from build123d import *

# Parameters (mm, degrees)
F0_R     = 6.45
F0_R_2   = 11.175
F1_DEPTH = 7
F2_R     = 3


with BuildPart() as f1:
    # F0 (on Top) → F1 (new body)
    with BuildSketch(Plane.XY):
        with BuildLine():
            ThreePointArc((9.599923, 11.660709), (13.65884, 6.447227), (15.103995, 0))
            ThreePointArc((15.103995, 0), (13.65884, -6.447227), (9.599923, -11.660709))
            ThreePointArc((9.599923, -11.660709), (14.033897, -12.989573), (18.629101, -13.546434))
            ThreePointArc((18.629101, -13.546434), (32.744063, -10.165399), (43.103995, 0))
            ThreePointArc((43.103995, 0), (32.744063, 10.165399), (18.629101, 13.546434))
            ThreePointArc((18.629101, 13.546434), (14.033897, 12.989573), (9.599923, 11.660709))
        make_face()
        with Locations((28.517951, 0)):
            Circle(F0_R, mode=Mode.SUBTRACT)
        with BuildLine():
            ThreePointArc((-9.599923, 11.660709), (0, 15.103995), (9.599923, 11.660709))
            ThreePointArc((9.599923, 11.660709), (14.033897, 12.989573), (18.629101, 13.546434))
            ThreePointArc((18.629101, 13.546434), (7.362471, 16.703494), (0, 25.797338))
            ThreePointArc((0, 25.797338), (-7.362471, 16.703494), (-18.629101, 13.546434))
            ThreePointArc((-18.629101, 13.546434), (-14.033897, 12.989573), (-9.599923, 11.660709))
        make_face()
        with BuildLine():
            ThreePointArc((18.629101, -13.546434), (14.033897, -12.989573), (9.599923, -11.660709))
            ThreePointArc((9.599923, -11.660709), (0, -15.103995), (-9.599923, -11.660709))
            ThreePointArc((-9.599923, -11.660709), (-14.033897, -12.989573), (-18.629101, -13.546434))
            ThreePointArc((-18.629101, -13.546434), (-7.362471, -16.703494), (0, -25.797338))
            ThreePointArc((0, -25.797338), (7.362471, -16.703494), (18.629101, -13.546434))
        make_face()
        with BuildLine():
            ThreePointArc((-9.599923, -11.660709), (-15.103995, 0), (-9.599923, 11.660709))
            ThreePointArc((-9.599923, 11.660709), (-14.033897, 12.989573), (-18.629101, 13.546434))
            ThreePointArc((-18.629101, 13.546434), (-32.744063, 10.165399), (-43.103995, 0))
            ThreePointArc((-43.103995, 0), (-32.744063, -10.165399), (-18.629101, -13.546434))
            ThreePointArc((-18.629101, -13.546434), (-14.033897, -12.989573), (-9.599923, -11.660709))
        make_face()
        with Locations((-28.517951, 0)):
            Circle(F0_R, mode=Mode.SUBTRACT)
        with BuildLine():
            ThreePointArc((9.599923, -11.660709), (13.65884, -6.447227), (15.103995, 0))
            ThreePointArc((15.103995, 0), (13.65884, 6.447227), (9.599923, 11.660709))
            ThreePointArc((9.599923, 11.660709), (0, 15.103995), (-9.599923, 11.660709))
            ThreePointArc((-9.599923, 11.660709), (-15.103995, 0), (-9.599923, -11.660709))
            ThreePointArc((-9.599923, -11.660709), (0, -15.103995), (9.599923, -11.660709))
        make_face()
        Circle(F0_R_2, mode=Mode.SUBTRACT)
    extrude(amount=F1_DEPTH)

    # F2
    f2_edges = [f1.edges().sort_by_distance(p)[0] for p in [
        (7.362471, -16.703494, 7),
        (32.744063, -10.165399, 7),
        (32.744063, 10.165399, 7),
        (7.362471, 16.703494, 7),
        (-7.362471, 16.703494, 7),
        (-32.744063, -10.165399, 7),
        (-7.362471, -16.703494, 7),
        (-32.744063, 10.165399, 7),
        (7.362471, -16.703494, 0),
        (32.744063, -10.165399, 0),
        (-7.362471, -16.703494, 0),
        (-32.744063, -10.165399, 0),
        (-32.744063, 10.165399, 0),
        (-7.362471, 16.703494, 0),
        (7.362471, 16.703494, 0),
        (32.744063, 10.165399, 0),
    ]]
    fillet(f2_edges, radius=F2_R)


solid = f1.part
Geometry: final body of the model. Coordinates: model frame, mm. Round coordinates to 2 decimals unless told otherwise and drop trailing zeros. Loops run counter-clockwise (first coordinate to the right, second up) from the corner with the lowest first, then second, coordinate; pieces in that order, holes last. Notation, with made-up numbers: (37, 17) -> (72, 17) arc R11 cw to (72, 24) -> close; hole circle Ø4 at (69, 12.5). An arc over 180 degrees is marked (long way). One line per question, with ' | ' between items. Start each with the question number.
1. Section A-A on z = 1.25. Output: boundary loops of the cut face in (x, y) (3 decimals).
2. Line query: line 1 along X through (y, z) = (0.5, 6.25); line 2 along Y through (x, z) = (-24, 1.5); line 3 along Y through (x, z) = (31, 6.25). Output: solid intervals per line, ascending. Write a range as [from, to].
3. Contact query for flat-ended pins moving along their axis: pin 1 (1.5 mm diameter, centred on y = -17.5, z = 1, fed in from -X); pin 2 (2 mm diameter, centred on y = 6.5, z = 6, fed in from -X); pin 3 (12 mm diameter, centred on x = -1, y = 9, fed in from -Z); pin 4 (2 mm diameter, centred on x = 25, z = 5.5, fed in from -Y). Output: stop coordinate, or through.
4. Mould query, pull axis Y, two halves, no side actions, for faces 1 (the face through (22.074, 0.284, 3.451)), 2 (the face through (7.502, 16.613, 3.493)), 3 (the face through (-9, -7, 0)), 4 (the face through (-7.502, -16.613, 3.493)). Classes: pulls with the +Y half, pulls with the -Y half, needs draft (parallel to the pull), parting line crosses it, or undercut.
5. Section B-B on y = 5. Count the separate pieces of the cut face and the enclosed holes in it, and give its area (3 significant figures).
Returned:
1) outline: (-42.451, 0) arc R26.604 ccw to (-18.649, -12.983) arc R19.831 cw to (0, -24.371) arc R19.831 cw to (18.649, -12.983) arc R26.604 ccw to (42.451, 0) arc R26.604 ccw to (18.649, 12.983) arc R19.831 cw to (0, 24.371) arc R19.831 cw to (-18.649, 12.983) arc R26.604 ccw to start; hole circle Ø12.9 at (-28.518, 0); hole circle Ø22.35 at (0, 0); hole circle Ø12.9 at (28.518, 0)
2) line 1: x = [-41.61, -34.95], [-22.09, -11.16], [11.16, 22.09], [34.95, 41.61] | line 2: y = [-12.8, -4.6], [4.6, 12.8] | line 3: y = [-9.93, -5.95], [5.95, 9.93]
3) pin 1: stops at x = -6.32 | pin 2: stops at x = -38.21 | pin 3: stops at z = 0 | pin 4: stops at y = -13.05
4) face 1: undercut | face 2: pulls with the +Y half | face 3: needs draft | face 4: pulls with the -Y half
5) separate pieces: 4 | enclosed holes: 0 | area: 287 mm2
